```python
from build123d import *

# Parameters (mm, degrees)
SKETCH_1_R           = 0.85
EXTRUDE_1_DEPTH      = 5
EXTRUDE_1_2_DEPTH    = 5
EXTRUDE_2_DEPTH      = 10
EXTRUDE_3_DEPTH      = 10
EXTRUDE_3_DEPTH_BACK = 10
SKETCH_3_W           = 4.9
SKETCH_3_H           = 5
FILLET_1_R           = 10


with BuildPart() as part:
    # Sketch 1 → Extrude 1 (new body)
    with BuildSketch(Plane(origin=(0, 0, 0), x_dir=(1, 0, 0), z_dir=(0, 1, 0))):
        with BuildLine():
            Line((-24, 10.5), (-24, -10.5))
            ThreePointArc((-24, -10.5), (-21, -13.5), (-18, -10.5))
            Line((-18, -10.5), (-18, 10.5))
            ThreePointArc((-18, 10.5), (-21, 13.5), (-24, 10.5))
        make_face()
        with Locations(Location((-21, 10.5, 0), (0, 0, 270))):
            Circle(SKETCH_1_R, mode=Mode.SUBTRACT)
        with Locations(Location((-21, -10.5, 0), (0, 0, 270))):
            Circle(SKETCH_1_R, mode=Mode.SUBTRACT)
    extrude(amount=EXTRUDE_1_DEPTH)



with BuildPart() as body_2:
    # Sketch 1 → Extrude 1 2 (new body)
    with BuildSketch(Plane(origin=(0, 0, 0), x_dir=(1, 0, 0), z_dir=(0, 1, 0))):
        with BuildLine():
            Line((24, -10.5), (24, 10.5))
            ThreePointArc((24, 10.5), (21, 13.5), (18, 10.5))
            Line((18, 10.5), (18, -10.5))
            ThreePointArc((18, -10.5), (21, -13.5), (24, -10.5))
        make_face()
        with Locations(Location((21, -10.5, 0), (0, 0, 270))):
            Circle(SKETCH_1_R, mode=Mode.SUBTRACT)
        with Locations(Location((21, 10.5, 0), (0, 0, 270))):
            Circle(SKETCH_1_R, mode=Mode.SUBTRACT)
    extrude(amount=EXTRUDE_1_2_DEPTH)


with BuildPart() as part_1:
    add(part.part)

    add(body_2.part)  # Extrude 2 merges body 2
    # Sketch 2 → Extrude 2 (add, symmetric)
    with BuildSketch(Plane.XY):
        Polygon((-18, 5), (-18, 0), (18, 0), (18, 5), (10, 13.8), (-10, 13.8), align=None)
    extrude(amount=EXTRUDE_2_DEPTH, both=True)

    # Sketch 3 → Extrude 3 (add, two sides: drawn at the far end of the back side and taken through both)
    with BuildSketch(Plane.XY.offset(-EXTRUDE_3_DEPTH_BACK)):
        with Locations((-7.55, 16.3)):
            Rectangle(SKETCH_3_W, SKETCH_3_H)
        with Locations((7.55, 16.3)):
            Rectangle(SKETCH_3_W, SKETCH_3_H)
    extrude(amount=EXTRUDE_3_DEPTH + EXTRUDE_3_DEPTH_BACK)

    # Fillet 1
    fillet_1_edges = [part_1.edges().sort_by_distance(p)[0] for p in [
        (-10, 13.8, 0),
        (10, 13.8, 0),
    ]]
    fillet(fillet_1_edges, radius=FILLET_1_R)


solid = part_1.part
```
Can you work these out from the model? Positions are in its coordinate system, mm. A direction names the side the tool comes from. Coordinates: 2 decimals unless noted, no trailing zeros. Loops run counter-clockwise (first coordinate to the right, second up) from the corner with the lowest first, then second, coordinate; pieces in that order, holes last.
1) Imagine slicing it at D-D on x = 1.5. List the corners of the cut face in (y, z) for me.
2) Which directions (+Z, -Z, +X, -X, +Y, -Y) give clear straight access to the entire face, cutting with the end or side of a thin tool? Please do faces 4 (the flat face through (-21, 5, 0)), 5 (the flat face through (5.1, 16, 0)), 6 (the flat face through (21, 5, 0)), 7 (the flat face through (0, 7, 10)).
3) Imagine slicing it at B-B on z = 3.75. List the corners of the cut face in (x, y) for me, plus the area to 3 significant figures.
4) Thinking about a two-plate mould opening in X: for faces 1 (the flat face through (-24, 2, 0)), 2 (the flat face through (0, 0, 0)), 3 (the cylindrical face through (20.246, 2.465, 10.892)), which applies, pulls with the +X half, pulls with the -X half, needs draft (parallel to the pull), parting line crosses it, or undercut?
5) Imagine slicing it at C-C on y = 16.25. List the corners of the cut face in (x, z) for me, plus the area to 3 significant figures.
6) Imagine slicing it at A-A on x = 21. List the corners of the cut face in (y, z) for me.
7) I need wall thicknesses on probe 1 along X at (y, z) = (3.6, 10.5); probe 2 along Y at (x, z) = (20, -7.5); probe 3 along Z at (x, y) = (8, 3). Which ranges of each line are inside material? Lowest first, please.
8) For pin 1 (5 mm diameter, centred on x = -1.5, z = 1, fed in from +Y); pin 2 (1 mm diameter, centred on x = -21, z = 10.5, fed in from +Y); pin 3 (0.6 mm diameter, centred on y = 18, z = 4.5, fed in from +X); pin 4 (5 mm diameter, centred on y = 15.5, z = -2.5, fed in from +X), each with a flat end and sliding along its axis, tell me the tip position at first contact or that it passes through.
Completed:
1. outline: (0, -10) - (13.8, -10) - (13.8, 10) - (0, 10) - close
2. face 4: +Z, -Z, -X, +Y
2. face 5: +Z, -Z, +Y
2. face 6: +Z, -Z, +X, +Y
2. face 7: +Z, +Y, -Y
3. outline: (-24, 0) - (24, 0) - (24, 5) - (18, 5) - (12.6, 10.94) arc R10 cw to (10, 17.67) - (10, 18.8) - (5.1, 18.8) - (5.1, 13.8) - (-5.1, 13.8) - (-5.1, 18.8) - (-10, 18.8) - (-10, 17.67) arc R10 cw to (-12.6, 10.94) - (-18, 5) - (-24, 5) - close
3. area: 539 mm2
4. face 1: pulls with the -X half
4. face 2: needs draft
4. face 3: undercut
5. outline: (-10.1, -10) - (-5.1, -10) - (-5.1, 10) - (-10.1, 10) - close; (5.1, -10) - (10.1, -10) - (10.1, 10) - (5.1, 10) - close
5. area: 200 mm2
6. outline: (0, -13.5) - (5, -13.5) - (5, -11.35) - (0, -11.35) - close; (0, -9.65) - (5, -9.65) - (5, 9.65) - (0, 9.65) - close; (0, 11.35) - (5, 11.35) - (5, 13.5) - (0, 13.5) - close
7. probe 1: x = -24 to -21.85, -20.15 to -18, 18 to 20.15, 21.85 to 24
7. probe 2: y = 0 to 5
7. probe 3: z = -10 to 10
8. pin 1: stops at y = 13.8
8. pin 2: passes through
8. pin 3: stops at x = 10
8. pin 4: stops at x = 11.16
